For this review, take the finished solid that the model builds, in its own axes (mm). Coordinates: 2 decimals unless noted, no trailing zeros. Order: outer loops, then holes, each group sorted by start corner. A loop starts at its lowest first (then second) coordinate and runs counter-clockwise, first axis right, second up.
Autodesk Inventor part; units mm, degrees
ref_plane "YZ Plane" through (0, 0, 0) normal (1, 0, 0) x (0, 1, 0)
ref_plane "XZ Plane" through (0, 0, 0) normal (0, 1, 0) x (-1, 0, 0)
ref_plane "XY Plane" through (0, 0, 0) normal (0, 0, 1) x (1, 0, 0)
sketch "Schizzo1" plane through (0, 0, 0) normal (1, 0, 0) x (0, 1, 0)
  line L0 (2.5344, 4.1858) -> (-5.3178, 4.1858)
  line L1 (-5.3178, -5.8142) -> (2.5344, -5.8142)
  line L2 (2.5344, -5.8142) -> (2.5344, 4.1858)
  circle A0 centre (-0.8257, -0.8142) radius 3
  line L3 (2.5344, 4.1858) -> (2.5344, -0.8142)
  arc A1 (-5.3178, 4.1858) -> (-5.3178, -5.8142) centre (8.3421, -0.8142) ccw
  point P0 (0, 0)
  dimension "d0" = 10
  dimension "d1" = 6
extrude "Estrusione1" add sketch "Schizzo1" against normal blind 5
thread "Filettatura1"
properties part number "porta vite senza fine"
1. Clearance check with a flat-ended pin moving along its axis: pin 1 Ø1.5 at (x, z) = (-3.5, 3) entering from -Y. State where the tip first meets the part, or that it passes through.
Answer below:
pin 1: stops at y = -5.88
2. The part is to be moulded in two halves that separate along Y. For faces 1 (the face through (-2.465, -6.204, -0.743)), 2 (the face through (-2.46, -1.48, -3.74)), 3 (the face through (0, -4, -1)), 4 (the face through (-2, 2.534, -1)), say which applies: +Y half, -Y half, draft (parallel to the pull), parting line (faces both ways), or undercut.
Answer below:
face 1: -Y half
face 2: undercut
face 3: draft
face 4: +Y half
3. To check wall thickness, follow L1, parallel to Z at x = -2.7, y = -1.5; L2, parallel to Y at x = -3.25, z = -2.5; L3, parallel to Z at x = -3.75, y = -2.5. State the ranges of each line that lie inside material, in increasing order.
Answer below:
L1: z = -5.81 to -3.74, 2.11 to 4.19
L2: y = -6.11 to -3.31, 1.66 to 2.53
L3: z = -5.81 to -3.3, 1.68 to 4.19
4. Take a section at C-C, the plane x = -4.55. Give the boundary of the cut face in (y, z), plus the area to 3 significant figures.
Answer below:
outline: (-5.32, -5.81) - (2.53, -5.81) - (2.53, 4.19) - (-5.32, 4.19) arc R14.55 ccw to start; hole circle Ø6 at (-0.83, -0.81)
area: 56.2 mm2
5. Take a section at D-D, the plane z = 2.75. Give the boundary of the cut face in (x, y).
Answer below:
outline: (-5, -5.76) - (0, -5.76) - (0, 2.53) - (-5, 2.53) - close
6. Take a section at A-A, the plane y = -0.5. Give the boundary of the cut face in (x, z), plus the area to 3 significant figures.
Answer below:
outline: (-5, -5.81) - (0, -5.81) - (0, -3.8) - (-5, -3.8) - close; (-5, 2.17) - (0, 2.17) - (0, 4.19) - (-5, 4.19) - close
area: 20.2 mm2
7. Take a section at B-B, the plane z = 1.5. Give the boundary of the cut face in (x, y).
Answer below:
outline: (-5, -6.02) - (0, -6.02) - (0, -2.73) - (-5, -2.73) - close; (-5, 1.08) - (0, 1.08) - (0, 2.53) - (-5, 2.53) - close
